Drawing for the job (mm, zero at the part's lowest x, y, z). Give positions to 0.01 mm unless a question says otherwise; leave off trailing zeros. Order: outer loops, then holes, each group sorted by start corner. A loop starts at its lowest first (then second) coordinate and runs counter-clockwise, first axis right, second up. Notation, with made-up numbers: (9, 62) - (39, 62) arc R17 ccw to (39, 72) - close; hole circle Ø5 at (-39, 1.25). An arc over 180 degrees is marked (long way). Use a Markdown table: item, result. Add a question column.
(1) Slice it at A-A (x = 16.45). Write the cut outline in (y, z), then the cut area to 3 significant figures.
(2) Flat gauge pins, fed straight in: pin 1 (4 mm diameter, centred on x = 21.22, z = 4.92, fed in from +Y); pin 2 (4 mm diameter, centred on x = 6.55, z = 24.04, fed in from -Y). Where does each tip first touch, or does it go through?
(3) Mould opens along Z. For the marked faces 1, 2 and 3 say: +Z half, -Z half, draft (parallel to the pull), parting line (faces both ways), or undercut.
(4) Slice it at D-D (x = 26). Write the cut outline in (y, z).
(5) Slice it at C-C (y = 2). Count the separate pieces of the cut face and the enclosed holes in it.
(6) Wall check: line 1 (Z direction, x = 19, y = 1.65); line 2 (Z direction, x = 6, y = 1.4) (1 decimal); line 3 (Z direction, x = 18.5, y = 1.25). Give the ranges that are in metal, low to high.
(7) Slice it at B-B (z = 16.45). Write the cut outline in (x, y), then the cut area to 3 significant figures.
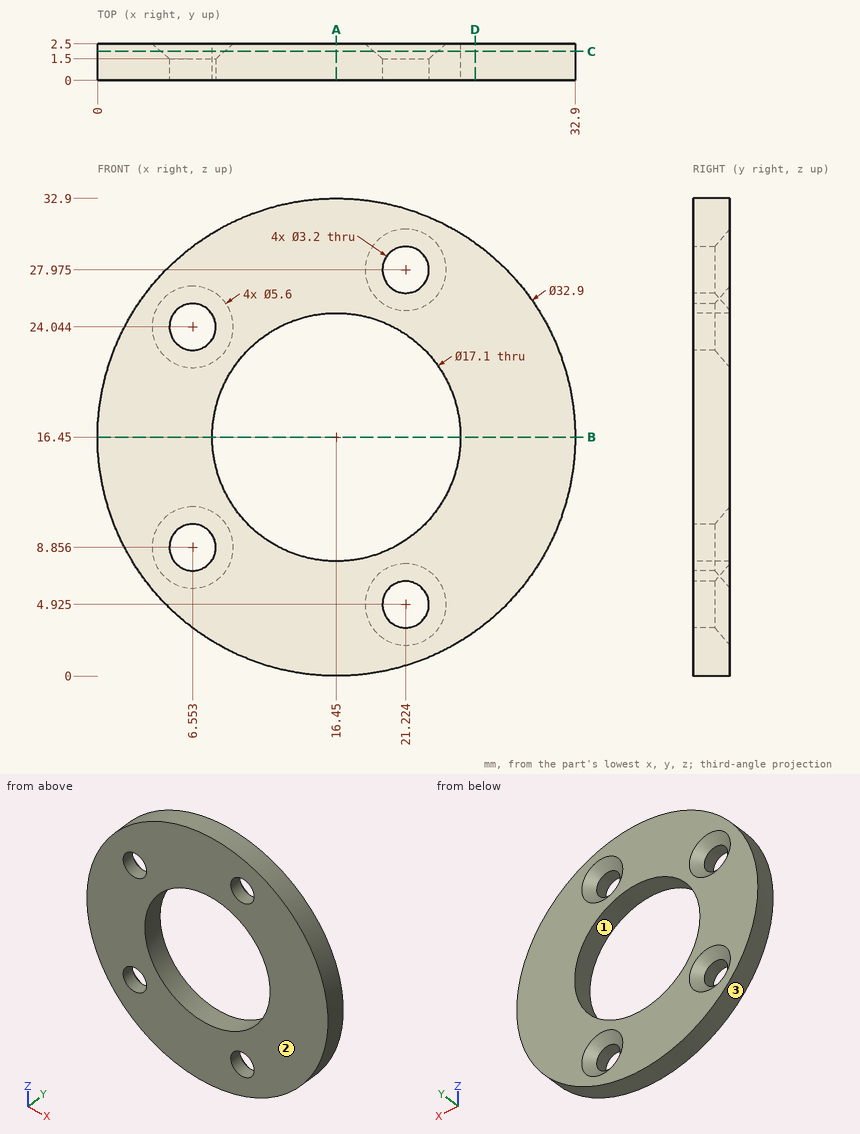
Solution:
| question | item | result |
|---|---|---|
| 1 | outline | (0, 0) - (2.5, 0) - (2.5, 7.9) - (0, 7.9) - close; (0, 25) - (2.5, 25) - (2.5, 32.9) - (0, 32.9) - close |
| 1 | area | 39.5 mm2 |
| 2 | pin 1 | y = 1.84 |
| 2 | pin 2 | y = 0 |
| 3 | face 1 | undercut |
| 3 | face 2 | draft |
| 3 | face 3 | parting line |
| 4 | outline | (0, 3.06) - (2.5, 3.06) - (2.5, 29.84) - (0, 29.84) - close |
| 5 | separate pieces | 1 |
| 5 | enclosed holes | 5 |
| 6 | line 1 | 0.2 to 8.29, 24.61 to 32.7 |
| 6 | line 2 | 3.7 to 7.4, 10.4 to 22.5, 25.5 to 29.2 |
| 6 | line 3 | 0.13 to 8.15, 24.75 to 32.77 |
| 7 | outline | (0, 0) - (7.9, 0) - (7.9, 2.5) - (0, 2.5) - close; (25, 0) - (32.9, 0) - (32.9, 2.5) - (25, 2.5) - close |
| 7 | area | 39.5 mm2 |
